Build history of the part. All positions in model axes, mm. Face numbers are marked on the shaded views. A direction names the side the tool comes from. Give positions to 0.01 mm unless a question says otherwise; leave off trailing zeros. Write each loop counter-clockwise with the first axis right and the second up, starting at its lowest first coordinate (ties: lowest second). Pieces come first, ordered by that corner, then holes. Notation, with made-up numbers: (14.25, 13.5) -> (33.25, 13.5) arc R32 ccw to (33.25, 51.5) -> close; hole circle Ø10 at (-23, 50.5). An arc over 180 degrees is marked (long way). Write item = value, one per line. Start each with the question number.
Q1. Saw through at A-A, the plane x = 0. List the corners of the cut face in (y, z).
Q2. Saw through at D-D, the plane y = -3.5. List the corners of the cut face in (x, z).
Q3. Tool access for the marked faces 1 and 2: list every direction of +Z, -Z, +X, -X, +Y, -Y with a clear straight run to the whole face (end or side of a thin tool).
Q4. Saw through at B-B, the plane y = 1.75. List the corners of the cut face in (x, z).
Q5. Drop flat-ended pins along their axis: P1, Ø2, axis at x = -0.5, z = -7.5, coming from the -Y side; P2, Ø5, axis at x = 0, y = 0, coming from the +Z side; P3, Ø2, axis at x = -4.5, z = -0.5, coming from the -Y side; P4, Ø1.5, axis at x = 2, y = 7, coming from the -Z side. Give the stop position or say it passes through.
Q6. Wall check: line 1 (Y direction, x = 0, z = -3.25); line 2 (Y direction, x = -3, z = -2.75); line 3 (Z direction, x = -3.75, y = -3.75). Give the ranges that are in metal, low to high.
Q7. Saw through at C-C, the plane z = -3.25. List the corners of the cut face in (x, y).
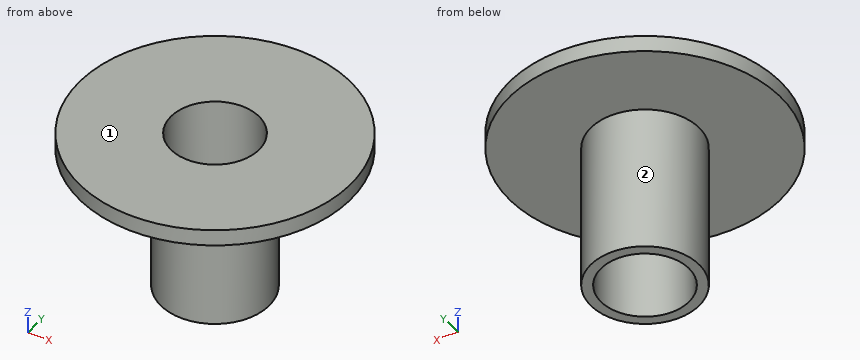
Autodesk Inventor part; units mm, degrees
ref_plane "YZ Plane" through (0, 0, 0) normal (1, 0, 0) x (0, 1, 0)
ref_plane "XZ Plane" through (0, 0, 0) normal (0, 1, 0) x (-1, 0, 0)
ref_plane "XY Plane" through (0, 0, 0) normal (0, 0, 1) x (1, 0, 0)
sketch "草圖1" plane through (0, 0, 0) normal (0, 0, 1) x (1, 0, 0)
  circle A0 centre (0, 0) radius 10
  dimension "d0" = 20
extrude "擠出1" add sketch "草圖1" along normal blind 1.2
sketch "草圖2" plane through (0, 0, 0) normal (0, 0, -1) x (-1, 0, 0)
  circle A0 centre (0, 0) radius 4
  dimension "d4" = 8
extrude "擠出2" cut sketch "草圖2" against normal up to next
sketch "草圖3" plane through (0, 0, 1.2) normal (0, 0, 1) x (1, 0, 0)
  circle A0 centre (0, 0) radius 4
  dimension "d7" = 8
extrude "擠出3" add sketch "草圖3" against normal blind 12
sketch "草圖4" plane through (0, 0, -10.8) normal (0, 0, -1) x (-1, 0, 0)
  circle A0 centre (0, 0) radius 3.25
  dimension "d10" = 6.5
extrude "擠出4" cut sketch "草圖4" against normal up to next
properties part number "儀表鐵軸套"
Report:
q1.outline = (-10, 0) -> (-4, 0) -> (-4, -10.8) -> (-3.25, -10.8) -> (-3.25, 1.2) -> (-10, 1.2) -> close; (3.25, -10.8) -> (4, -10.8) -> (4, 0) -> (10, 0) -> (10, 1.2) -> (3.25, 1.2) -> close
q2.outline = (-9.37, 0) -> (-1.94, 0) -> (-1.94, -10.8) -> (1.94, -10.8) -> (1.94, 0) -> (9.37, 0) -> (9.37, 1.2) -> (-9.37, 1.2) -> close
q3.face_1 = +Z, +X, -X, +Y, -Y
q3.face_2 = -Z
q4.outline = (-9.85, 0) -> (-3.6, 0) -> (-3.6, -10.8) -> (-2.74, -10.8) -> (-2.74, 1.2) -> (-9.85, 1.2) -> close; (2.74, -10.8) -> (3.6, -10.8) -> (3.6, 0) -> (9.85, 0) -> (9.85, 1.2) -> (2.74, 1.2) -> close
q5.P1 = -4
q5.P2 = through
q5.P3 = -9.32
q5.P4 = 0
q6.line_1 = -4 to -3.25, 3.25 to 4
q6.line_2 = -2.65 to -1.25, 1.25 to 2.65
q6.line_3 = 0 to 1.2
q7.outline = circle Ø8 at (0, 0); hole circle Ø6.5 at (0, 0)
